Input: part model. Units: mm. Frame: model coordinates. A direction names the side the tool comes from. Coordinates: 2 decimals unless noted, no trailing zeros. Write each loop counter-clockwise with the first axis right and the second up, starting at its lowest first coordinate (ties: lowest second). Pieces come first, ordered by that corner, then holes. Notation, with made-up numbers: (29.5, 18) - (47.5, 18) arc R35 cw to (47.5, 56) - close; hole circle Ø3 at (39.25, 81.5). An arc over 180 degrees is marked (long way). Use CSV: the item, a comma, the result in double quotes.
```python
from build123d import *

# Parameters (mm, degrees)
SKETCH_1_R          = 12.5
EXTRUDE_1_DEPTH     = 30
SKETCH_4_R          = 1.5
CUT_EXTRUDE_1_DEPTH = 0.5
SKETCH_3_W          = 6
SKETCH_3_H          = 6
EXTRUDE_2_DEPTH     = 4


with BuildPart() as part:
    # 草图1 → 凸台-拉伸1 (new body)
    with BuildSketch(Plane.XY):
        Circle(SKETCH_1_R)
    extrude(amount=EXTRUDE_1_DEPTH)

    # 草图4 → 切除-拉伸1 (cut)
    with BuildSketch(Plane(origin=(0, 0, 0), x_dir=(-1, 0, 0), z_dir=(0, 0, -1))):
        with Locations((-8.5, 0)):
            Circle(SKETCH_4_R)
        with Locations(Location((8.5, 0, 0), (0, 0, 180))):
            Circle(SKETCH_4_R)
    extrude(amount=-CUT_EXTRUDE_1_DEPTH, mode=Mode.SUBTRACT)

    # 草图2 → 旋转2 (revolve)
    with BuildSketch(Plane(origin=(0, 0, 0), x_dir=(1, 0, 0), z_dir=(0, 1, 0))):
        Polygon((5, 28), (0, 28), (0, 0), (0.75, 0), (0.75, 5), (5, 5), (5, 26), (7.5, 26), (7.5, 28), align=None)
    revolve(axis=Axis((0, 0, 1000), (0, 0, -1)))

    # 草图3 → 凸台-拉伸2 (add)
    with BuildSketch(Plane(origin=(0, 0, -28), x_dir=(-1, 0, 0), z_dir=(0, 0, -1))):
        Rectangle(SKETCH_3_W, SKETCH_3_H)
    extrude(amount=EXTRUDE_2_DEPTH)


solid = part.part
```
(1) Cut plane D-D on y = 6. Return loops of the section in (x, z), and give its area (3 significant figures).
Check values:
outline,"(-10.97, 0) - (10.97, 0) - (10.97, 30) - (-10.97, 30) - close; (-4.5, -28) - (4.5, -28) - (4.5, -26) - (-4.5, -26) - close"
area,"676 mm^2"
(2) Cut plane B-B on x = -1.5. Return loops of the section in (y, z).
Check values:
outline,"(-12.41, 0) - (12.41, 0) - (12.41, 30) - (-12.41, 30) - close; (-7.35, -28) - (-3, -28) - (-3, -32) - (3, -32) - (3, -28) - (7.35, -28) - (7.35, -26) - (4.77, -26) - (4.77, -5) - (-4.77, -5) - (-4.77, -26) - (-7.35, -26) - close"
(3) Draft query along Z for faces 1 (the flat face through (0, 0, -32)), 2 (the flat face through (0, 3, -30)), 3 (the cylindrical face through (10, 0.07, 0.25)). Return one class per face: pulls with the +Z half, pulls with the -Z half, needs draft (parallel to the pull), parting line crosses it, or undercut.
Check values:
face 1,"pulls with the -Z half"
face 2,"needs draft"
face 3,"undercut"
(4) Cut plane C-C on x = -8.25. Return loops of the section in (y, z).
Check values:
outline,"(-9.39, 0) - (-1.48, 0) - (-1.48, 0.5) - (1.48, 0.5) - (1.48, 0) - (9.39, 0) - (9.39, 30) - (-9.39, 30) - close"
(5) Pin query (flat end, axial travel): pin 1 Ø1.5 at (x, y) = (-8, -0.5) entering from -Z; pin 2 Ø4.5 at (y, z) = (0.5, -31) entering from +X; pin 3 Ø2 at (y, z) = (5.5, 4.5) entering from +X. Return the tip coordinate at first contact, or that it passes through.
Check values:
pin 1,"z = -28"
pin 2,"x = 3"
pin 3,"x = 11.66"
(6) Cut plane A-A on y = 0. Return loops of the section in (x, z).
Check values:
outline,"(-12.5, 0) - (-10, 0) - (-10, 0.5) - (-7, 0.5) - (-7, 0) - (-0.75, 0) - (-0.75, -5) - (-5, -5) - (-5, -26) - (-7.5, -26) - (-7.5, -28) - (-3, -28) - (-3, -32) - (3, -32) - (3, -28) - (7.5, -28) - (7.5, -26) - (5, -26) - (5, -5) - (0.75, -5) - (0.75, 0) - (7, 0) - (7, 0.5) - (10, 0.5) - (10, 0) - (12.5, 0) - (12.5, 30) - (-12.5, 30) - close"
(7) Ray query, probe 1 along Z at (x, y) = (-3.5, 2.25); probe 2 along Z at (x, y) = (-5.5, -0.25); probe 3 along Z at (x, y) = (-10, 6.75). Return the intervals inside material, ascending. Write a range as from..to.
Check values:
probe 1,"-28..-5, 0..30"
probe 2,"-28..-26, 0..30"
probe 3,"0..30"
(8) Reachability of faces 4 (the flat face through (0, -3, -30)), 5 (the cylindrical face through (-7.493, -0.33, -27.014)), 6 (the cylindrical face through (-10, -0.07, 0.25)) from +Z, -Z, +X, -X, +Y, -Y: full face, straight path, thin tool, end or side. Return the list, or none.
Check values:
face 4,"-Z, +X, -X, -Y"
face 5,"-Z"
face 6,"none"
